from build123d import *

# Parameters (mm, degrees)
SKIZZE2_W                       = 217
SKIZZE2_H                       = 155
AUFSATZ_LINEAR_AUSTRAGEN1_DEPTH = 60
WANDUNG1_T                      = -5
SCHNITT_LINEAR_AUSTRAGEN1_REACH = 200.487
SKIZZE7_R                       = 1.5
SKIZZE8_W                       = 10
SKIZZE8_H                       = 10
AUFSATZ_LINEAR_AUSTRAGEN2_DEPTH = 10
SCHNITT_LINEAR_AUSTRAGEN2_REACH = 157.366
FASE1_SIZE                      = 3


with BuildPart() as part:
    # Skizze2 → Aufsatz-Linear austragen1 (new body)
    with BuildSketch(Plane(origin=(0, 0, 0), x_dir=(1, 0, 0), z_dir=(0, 1, 0))):
        Rectangle(SKIZZE2_W, SKIZZE2_H)
    extrude(amount=AUFSATZ_LINEAR_AUSTRAGEN1_DEPTH)

    # Wandung1
    wandung1_openings = [part.faces().sort_by_distance(p)[0] for p in [
        (0, 60, 0),
    ]]
    offset(amount=WANDUNG1_T, openings=wandung1_openings, kind=Kind.INTERSECTION)

    # Skizze7 → Schnitt-Linear austragen1 (cut, up to next)
    with BuildSketch(Plane.XY.offset(77.5), mode=Mode.PRIVATE) as schnitt_linear_austragen1_sk1:
        with Locations((-93.5, 55)):
            Circle(SKIZZE7_R)
    schnitt_linear_austragen1_tool1 = extrude(schnitt_linear_austragen1_sk1.sketch, amount=-SCHNITT_LINEAR_AUSTRAGEN1_REACH, mode=Mode.PRIVATE) & part.part
    # Skizze7 → Schnitt-Linear austragen1 (cut, up to next)
    with BuildSketch(Plane.XY.offset(77.5), mode=Mode.PRIVATE) as schnitt_linear_austragen1_sk2:
        with Locations((-78.5, 55)):
            Circle(SKIZZE7_R)
    schnitt_linear_austragen1_tool2 = extrude(schnitt_linear_austragen1_sk2.sketch, amount=-SCHNITT_LINEAR_AUSTRAGEN1_REACH, mode=Mode.PRIVATE) & part.part
    # Skizze7 → Schnitt-Linear austragen1 (cut, up to next)
    with BuildSketch(Plane.XY.offset(77.5), mode=Mode.PRIVATE) as schnitt_linear_austragen1_sk3:
        with Locations((78.5, 55)):
            Circle(SKIZZE7_R)
    schnitt_linear_austragen1_tool3 = extrude(schnitt_linear_austragen1_sk3.sketch, amount=-SCHNITT_LINEAR_AUSTRAGEN1_REACH, mode=Mode.PRIVATE) & part.part
    # Skizze7 → Schnitt-Linear austragen1 (cut, up to next)
    with BuildSketch(Plane.XY.offset(77.5), mode=Mode.PRIVATE) as schnitt_linear_austragen1_sk4:
        with Locations((93.5, 55)):
            Circle(SKIZZE7_R)
    schnitt_linear_austragen1_tool4 = extrude(schnitt_linear_austragen1_sk4.sketch, amount=-SCHNITT_LINEAR_AUSTRAGEN1_REACH, mode=Mode.PRIVATE) & part.part
    add(schnitt_linear_austragen1_tool1.solids().sort_by_distance((-93.5, 55, 77.5))[0], mode=Mode.SUBTRACT)
    add(schnitt_linear_austragen1_tool2.solids().sort_by_distance((-78.5, 55, 77.5))[0], mode=Mode.SUBTRACT)
    add(schnitt_linear_austragen1_tool3.solids().sort_by_distance((78.5, 55, 77.5))[0], mode=Mode.SUBTRACT)
    add(schnitt_linear_austragen1_tool4.solids().sort_by_distance((93.5, 55, 77.5))[0], mode=Mode.SUBTRACT)

    # Skizze8 → Aufsatz-Linear austragen2 (add)
    with BuildSketch(Plane.XY.offset(77.5)):
        with Locations((0, 55)):
            Rectangle(SKIZZE8_W, SKIZZE8_H)
    extrude(amount=AUFSATZ_LINEAR_AUSTRAGEN2_DEPTH)

    # Skizze9 → Schnitt-Linear austragen2 (cut, up to next)
    with BuildSketch(Plane.ZY.offset(5), mode=Mode.PRIVATE) as schnitt_linear_austragen2_sk1:
        Polygon((77.5, 50), (87.5, 60), (87.5, 50), align=None)
    schnitt_linear_austragen2_tool1 = extrude(schnitt_linear_austragen2_sk1.sketch, amount=-SCHNITT_LINEAR_AUSTRAGEN2_REACH, mode=Mode.PRIVATE) & part.part
    add(schnitt_linear_austragen2_tool1.solids().sort_by_distance((-5, 53.333333, 84.166667))[0], mode=Mode.SUBTRACT)

    # Fase1
    fase1_edges = [part.edges().sort_by_distance(p)[0] for p in [
        (103.5, 5, 0),
        (103.5, 32.5, 72.5),
        (0, 5, -72.5),
        (103.5, 32.5, -72.5),
        (-103.5, 32.5, -72.5),
        (-103.5, 32.5, 72.5),
        (0, 0, 77.5),
        (-108.5, 0, 0),
        (0, 0, -77.5),
        (108.5, 0, 0),
        (108.5, 30, 77.5),
        (-108.5, 30, 77.5),
        (-108.5, 30, -77.5),
        (108.5, 30, -77.5),
    ]]
    chamfer(fase1_edges, length=FASE1_SIZE)


solid = part.part
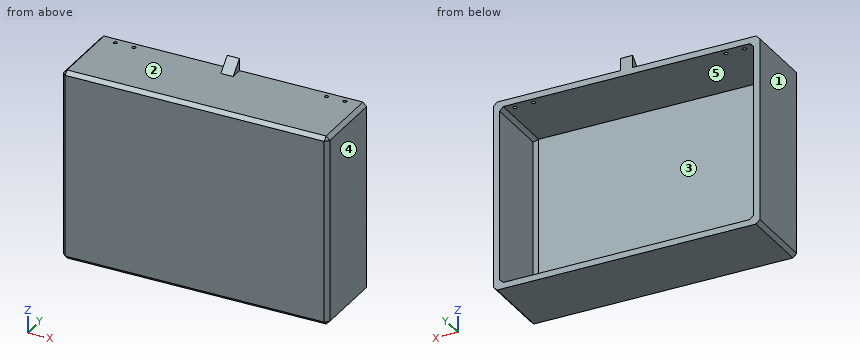
Part model, mm, in its own coordinate system. Face numbers are marked on the shaded views. A direction names the side the tool comes from. Give positions to 0.01 mm unless a question says otherwise; leave off trailing zeros. Order: outer loops, then holes, each group sorted by start corner. A loop starts at its lowest first (then second) coordinate and runs counter-clockwise, first axis right, second up. Notation, with made-up numbers: (72, 84.25) -> (116, 84.25) arc R30 ccw to (116, 116.25) -> close; hole circle Ø8 at (-14, 24.5). An arc over 180 degrees is marked (long way). Use one line per item in the form item = value.
(1) Saw through at B-B (x = 17). Write the cut outline in (y, z), then the cut area to 3 significant figures.
Solution:
outline = (0, -74.5) -> (3, -77.5) -> (60, -77.5) -> (60, -72.5) -> (8, -72.5) -> (5, -69.5) -> (5, 72.5) -> (60, 72.5) -> (60, 77.5) -> (3, 77.5) -> (0, 74.5) -> close
area = 1,320 mm²
(2) Drill centre lines: line 1 (Z direction, x = -75, y = 27.5); line 2 (X direction, y = 17, z = -9); line 3 (Y direction, x = -78.5, z = 74.05). Where is each one in solid material? Low to high. Write a range as from..to.
Solution:
line_1 = -77.5..-72.5, 72.5..77.5
line_2 = -108.5..-103.5, 103.5..108.5
line_3 = 0..53.5, 56.5..60
(3) Pull direction Z, two halves, no side cores. Call the marked faces 1, 2 and 3: +Z half, -Z half, draft (parallel to the pull), parting line (faces both ways), or undercut.
Solution:
face_1 = draft
face_2 = +Z half
face_3 = undercut
(4) Saw through at A-A (z = -59.5). Write the cut outline in (x, y), then the cut area to 3 significant figures.
Solution:
outline = (-108.5, 3) -> (-105.5, 0) -> (105.5, 0) -> (108.5, 3) -> (108.5, 60) -> (103.5, 60) -> (103.5, 8) -> (100.5, 5) -> (-103.5, 5) -> (-103.5, 60) -> (-108.5, 60) -> close
area = 1,630 mm²
(5) Tool access for the marked faces 4 and 5: list every direction of +Z, -Z, +X, -X, +Y, -Y with a clear straight run to the whole face (end or side of a thin tool).
Solution:
face_4 = +Z, -Z, +X, +Y, -Y
face_5 = +Y
(6) Flat gauge pins, fed straight in: P1, Ø1, axis at x = -27.5, y = 51, coming from the +Z side; P2, Ø5, axis at y = 55.5, z = 83, coming from the -X side; P3, Ø1, axis at x = -83.5, z = 49.5, coming from the +Y side. Where does each tip first touch, or does it go through?
Solution:
P1 = 77.5
P2 = -5
P3 = 5
